Work out the finished part from the listing and answer in its coordinate system (mm). Round coordinates to 2 decimals unless told otherwise and drop trailing zeros. Loops run counter-clockwise (first coordinate to the right, second up) from the corner with the lowest first, then second, coordinate; pieces in that order, holes last.
from build123d import *

# Parameters (mm, degrees)
SKETCH2_W           = 38.1
SKETCH2_H           = 101.6
SKETCH2_R           = 3.175
BOSS_EXTRUDE1_DEPTH = 6.35
SKETCH3_R           = 3.175
CUT_EXTRUDE2_DEPTH  = 7.35


with BuildPart() as part:
    # Sketch2 → Boss-Extrude1 (new body)
    with BuildSketch(Plane(origin=(0, 0, 0), x_dir=(1, 0, 0), z_dir=(0, 1, 0))):
        with Locations((6.35, 0)):
            Rectangle(SKETCH2_W, SKETCH2_H)
        Circle(SKETCH2_R, mode=Mode.SUBTRACT)
        with Locations((0, 38.1)):
            Circle(SKETCH2_R, mode=Mode.SUBTRACT)
        with Locations((0, -38.1)):
            Circle(SKETCH2_R, mode=Mode.SUBTRACT)
    extrude(amount=BOSS_EXTRUDE1_DEPTH)

    # Sketch3 → Cut-Extrude2 (cut, through all)
    with BuildSketch(Plane(origin=(0, 6.35, 0), x_dir=(1, 0, 0), z_dir=(0, 1, 0))):
        with Locations((18.58962745, 28.575)):
            Circle(SKETCH3_R)
        with Locations((18.58962745, 9.525)):
            Circle(SKETCH3_R)
        with Locations((18.58962745, -9.525)):
            Circle(SKETCH3_R)
        with Locations((18.58962745, -28.575)):
            Circle(SKETCH3_R)
    extrude(amount=-CUT_EXTRUDE2_DEPTH, mode=Mode.SUBTRACT)


solid = part.part
Item 1: Section D-D, the plane z = -8.5 is taken. Give the vertices of the cut face in (x, y).
Item 2: Determine the mould class of faces 1 (the face through (6, 3, 50.8)), 2 (the face through (6, 3, -50.8)), 3 (the face through (6, 6.35, -1)), 4 (the face through (-0.69, 3.13, -35)) for opening direction Z: pulls with the +Z half, pulls with the -Z half, needs draft (parallel to the pull), parting line crosses it, or undercut.
Item 3: Section B-B, the plane x = 0 is taken. Give the vertices of the cut face in (y, z) (3 decimals), plus the area to 3 significant figures.
Item 4: Section A-A, the plane z = -38.1 is taken. Give the vertices of the cut face in (x, y) (3 decimals), plus the area to 3 significant figures.
Item 5: Section C-C, the plane y = 1.5 is taken. Give the vertices of the cut face in (x, z) (3 decimals), plus the area to 3 significant figures.
Item 6: Straight lines are drawn through the part: line 1 (Z direction, x = 18.5, y = 0.5); line 2 (X direction, y = 3.5, z = -28.5); line 3 (Z direction, x = 0, y = 1.75) (3 decimals). For each, find the intervals that lie inside material, in ascending order.
Answer below:
1. outline: (-12.7, 0) - (15.58, 0) - (15.58, 6.35) - (-12.7, 6.35) - close; (21.59, 0) - (25.4, 0) - (25.4, 6.35) - (21.59, 6.35) - close
2. face 1: pulls with the +Z half
2. face 2: pulls with the -Z half
2. face 3: needs draft
2. face 4: undercut
3. outline: (0, -50.8) - (6.35, -50.8) - (6.35, -41.275) - (0, -41.275) - close; (0, -34.925) - (6.35, -34.925) - (6.35, -3.175) - (0, -3.175) - close; (0, 3.175) - (6.35, 3.175) - (6.35, 34.925) - (0, 34.925) - close; (0, 41.275) - (6.35, 41.275) - (6.35, 50.8) - (0, 50.8) - close
3. area: 524 mm2
4. outline: (-12.7, 0) - (-3.175, 0) - (-3.175, 6.35) - (-12.7, 6.35) - close; (3.175, 0) - (25.4, 0) - (25.4, 6.35) - (3.175, 6.35) - close
4. area: 202 mm2
5. outline: (-12.7, -50.8) - (25.4, -50.8) - (25.4, 50.8) - (-12.7, 50.8) - close; hole circle Ø6.35 at (0, -38.1); hole circle Ø6.35 at (0, 0); hole circle Ø6.35 at (0, 38.1); hole circle Ø6.35 at (18.59, -28.575); hole circle Ø6.35 at (18.59, -9.525); hole circle Ø6.35 at (18.59, 9.525); hole circle Ø6.35 at (18.59, 28.575)
5. area: 3,650 mm2
6. line 1: z = -50.8 to -31.75, -25.4 to -12.7, -6.35 to 6.35, 12.7 to 25.4, 31.75 to 50.8
6. line 2: x = -12.7 to 15.42, 21.76 to 25.4
6. line 3: z = -50.8 to -41.275, -34.925 to -3.175, 3.175 to 34.925, 41.275 to 50.8
